Model file for the job. Use its own axes, mm. A direction names the side the tool comes from. Round coordinates to 2 decimals unless told otherwise and drop trailing zeros. Write each loop counter-clockwise with the first axis right and the second up, starting at its lowest first coordinate (ties: lowest second). Pieces come first, ordered by that corner, then holes. Notation, with made-up numbers: (-11, 41.25) - (44, 41.25) arc R20 ccw to (44, 47.25) - close; hole circle Ø7 at (58, -20.75). An arc over 180 degrees is marked (long way). Answer as a JSON object with one key per item and string values. Group by question number.
from build123d import *

# Parameters (mm, degrees)
SKETCH1_W           = 1.524
SKETCH1_H           = 1.524
BOSS_EXTRUDE1_DEPTH = 1.524
CUT_EXTRUDE1_DEPTH  = 2.54
CUT_EXTRUDE2_DEPTH  = 2.54


with BuildPart() as part:
    # Sketch1 → Boss-Extrude1 (new body)
    with BuildSketch(Plane.XY):
        with BuildLine():
            ThreePointArc((-5.144991791, -6.632201856), (7.805780573, -0.762), (-5.144991791, 5.108201856))
            ThreePointArc((-5.144991791, 5.108201856), (-11.231180242, 3.023042691), (-17.599967494, 2.113027551))
            ThreePointArc((-17.599967494, 2.113027551), (-20.474995045, -0.762), (-17.599967494, -3.637027551))
            ThreePointArc((-17.599967494, -3.637027551), (-11.231180242, -4.547042691), (-5.144991791, -6.632201856))
        make_face()
        with Locations((0.762, -0.762)):
            Rectangle(SKETCH1_W, SKETCH1_H, mode=Mode.SUBTRACT)
    extrude(amount=-BOSS_EXTRUDE1_DEPTH)

    # Sketch2 → Cut-Extrude1 (cut)
    with BuildSketch(Plane.XY):
        Polygon((-9.141246891, -1.667471429), (-13.932743082, -4.156077978), (-13.230301809, -5.508539533), (-8.438805618, -3.019932984), align=None)
        Polygon((-13.932743082, 2.632077978), (-13.230301809, 3.984539533), (-8.438805618, 1.495932984), (-9.141246891, 0.143471429), align=None)
    extrude(amount=-CUT_EXTRUDE1_DEPTH, mode=Mode.SUBTRACT)

    # Sketch3 → Cut-Extrude2 (cut)
    with BuildSketch(Plane.XY):
        Polygon((1.03592119, 3.823335546), (1.390623256, 2.34118763), (-2.266113377, 1.466071171), (-2.620815442, 2.948219087), align=None)
        Polygon((-2.620815442, -4.472219087), (1.03592119, -5.347335546), (1.390623256, -3.86518763), (-2.266113377, -2.990071171), align=None)
    extrude(amount=-CUT_EXTRUDE2_DEPTH, mode=Mode.SUBTRACT)


solid = part.part
(1) 3-axis set-ups, long thin cutter, end or side, ignore diameter. For faces 4 (the flat face through (0, -1, -1)), 5 (the cylindrical face through (-20.474, -0.699, -0.751)): which of +Z, -Z, +X, -X, +Y, -Y reach the whole face in a straight line?
(2) Slice it at C-C (y = 6). Write the cut outline in (x, z), then the cut area to 3 significant figures.
(3) Flat gauge pin, fed straight in: pin 1 (0.5 mm diameter, centred on x = 0.5, z = -1, fed in from +Y). Where does the tip first touch, or does it go through?
(4) Pull direction Y, two halves, no side cores. Call faces 1 (the cylindrical face through (-15.681, -3.783, -0.751)), 2 (the flat face through (-3, -1, 0)), 3 (the flat face through (-9.906, -3.782, -0.751)): pulls with the +Y half, pulls with the -Y half, needs draft (parallel to the pull), parting line crosses it, or undercut.
(5) Slice it at D-D (x = -9.75). Write the cut outline in (y, z).
(6) Slice it at A-A (z = -0.75). Write the cut outline in (x, y) (3 decimals).
(7) Slice it at B-B (x = -1.25). Write the cut outline in (y, z), then the cut area to 3 significant figures.
(8) Drill centre lines: line 1 (Y direction, x = 1, z = -0.8); line 2 (X direction, y = 0.5, z = -0.75); line 3 (X direction, y = -0.5, z = -0.1). Where is each one in solid material? Low to high. Write a range as from..to.
Answer:
{
 "1": {"face 4": "+Z, -Z", "face 5": "+Z, -Z, -X"},
 "2": {"outline": "(-3.9, -1.52) - (3.9, -1.52) - (3.9, 0) - (-3.9, 0) - close", "area": "11.9 mm²"},
 "3": {"pin 1": "y = 7.04"},
 "4": {"face 1": "pulls with the -Y half", "face 2": "needs draft", "face 3": "undercut"},
 "5": {"outline": "(-4.94, -1.52) - (-3.7, -1.52) - (-3.7, 0) - (-4.94, 0) - close; (-1.98, -1.52) - (0.46, -1.52) - (0.46, 0) - (-1.98, 0) - close; (2.18, -1.52) - (3.41, -1.52) - (3.41, 0) - (2.18, 0) - close"},
 "6": {"outline": "(-17.6, -3.637) arc R34.245 cw to (-13.72, -4.045) - (-9.141, -1.667) - (-8.439, -3.02) - (-11.332, -4.523) arc R34.245 cw to (-5.145, -6.632) arc R7.806 ccw (long way) to (-5.145, 5.108) arc R34.245 cw to (-11.332, 2.999) - (-8.439, 1.496) - (-9.141, 0.143) - (-13.72, 2.521) arc R34.245 cw to (-17.6, 2.113) arc R2.875 ccw to start; hole (-2.621, -4.472) - (1.036, -5.347) - (1.391, -3.865) - (-2.266, -2.99) - close; hole (-2.621, 2.948) - (-2.266, 1.466) - (1.391, 2.341) - (1.036, 3.823) - close; hole (0, -1.524) - (1.524, -1.524) - (1.524, 0) - (0, 0) - close"},
 "7": {"outline": "(-8.47, -1.52) - (-4.8, -1.52) - (-4.8, 0) - (-8.47, 0) - close; (-3.23, -1.52) - (1.71, -1.52) - (1.71, 0) - (-3.23, 0) - close; (3.28, -1.52) - (6.94, -1.52) - (6.94, 0) - (3.28, 0) - close", "area": "18.7 mm²"},
 "8": {"line 1": "-8.5..-5.34, -3.77..-1.52, 0..2.25, 3.81..6.98", "line 2": "-20.18..-9.83, -8.96..7.7", "line 3": "-20.46..0, 1.52..7.8"}
}
